Check sheet for the modelled part. Datum: model origin and axes. Units: mm. A direction names the side the tool comes from. Round coordinates to 2 decimals unless told otherwise and drop trailing zeros. Write each loop counter-clockwise with the first axis right and the second up, starting at its lowest first coordinate (ties: lowest second). Pieces come first, ordered by that corner, then holes.
from build123d import *

# Parameters (mm, degrees)
SKETCH_1_R          = 17.4
EXTRUDE_1_DEPTH     = 30
SKETCH_2_R          = 13.5
CUT_EXTRUDE_1_DEPTH = 39.801030914
SKETCH_3_W          = 7.6
SKETCH_3_H          = 1.8
SKETCH_3_W_2        = 1.8
SKETCH_3_H_2        = 7.6
EXTRUDE_2_DEPTH     = 3
SKETCH_4_W          = 20
SKETCH_4_H          = 10
CUT_EXTRUDE_2_DEPTH = 42.164547854
FILLET_1_R          = 5
SKETCH_5_W          = 23.4
SKETCH_5_H          = 23.4
CUT_EXTRUDE_3_DEPTH = 5
FILLET_2_R          = 5


with BuildPart() as part:
    # 草图1 → 凸台-拉伸1 (new body)
    with BuildSketch(Plane(origin=(0, 0, 0), x_dir=(1, 0, 0), z_dir=(0, 1, 0))):
        with Locations(Location((0, 0, 0), (0, 0, 270))):
            Circle(SKETCH_1_R)
    extrude(amount=EXTRUDE_1_DEPTH)

    # 草图2 → 切除-拉伸1 (cut, through all)
    with BuildSketch(Plane(origin=(0, 30, 0), x_dir=(1, 0, 0), z_dir=(0, 1, 0))):
        with Locations(Location((0, 0, 0), (0, 0, 270))):
            Circle(SKETCH_2_R)
    extrude(amount=-CUT_EXTRUDE_1_DEPTH, mode=Mode.SUBTRACT)

    # 草图3 → 凸台-拉伸2 (add)
    with BuildSketch(Plane(origin=(0, 30, 0), x_dir=(1, 0, 0), z_dir=(0, 1, 0))):
        Polygon((13.7, 3.8), (13.7, 0), (13.7, -3.8), (15.5, -3.8), (15.5, 3.8), align=None)
        with Locations((0, -14.6)):
            Rectangle(SKETCH_3_W, SKETCH_3_H)
        with Locations((-14.6, 0)):
            Rectangle(SKETCH_3_W_2, SKETCH_3_H_2)
        with Locations((0, 14.6)):
            Rectangle(SKETCH_3_W, SKETCH_3_H)
    extrude(amount=EXTRUDE_2_DEPTH)

    # 草图4 → 切除-拉伸2 (cut, through all)
    with BuildSketch(Plane(origin=(0, 0, 0), x_dir=(0, 0, -1), z_dir=(1, 0, 0))):
        with Locations((0, 5)):
            Rectangle(SKETCH_4_W, SKETCH_4_H)
    extrude(amount=-CUT_EXTRUDE_2_DEPTH, mode=Mode.SUBTRACT)

    # 圆角1
    fillet_1_edges = [part.edges().sort_by_distance(p)[0] for p in [
        (-11.654280291, 10, -10),
        (-11.654280291, 10, 10),
    ]]
    fillet(fillet_1_edges, radius=FILLET_1_R)

    # 草图5 → 切除-拉伸3 (cut)
    with BuildSketch(Plane(origin=(0, 30, 0), x_dir=(1, 0, 0), z_dir=(0, 1, 0))):
        Rectangle(SKETCH_5_W, SKETCH_5_H)
    extrude(amount=-CUT_EXTRUDE_3_DEPTH, mode=Mode.SUBTRACT)

    # 圆角2
    fillet_2_edges = [part.edges().sort_by_distance(p)[0] for p in [
        (11.7, 27.5, -6.734983296),
        (11.7, 27.5, 6.734983296),
        (6.734983296, 27.5, 11.7),
        (-6.734983296, 27.5, 11.7),
        (-11.7, 27.5, 6.734983296),
        (-11.7, 27.5, -6.734983296),
        (-6.734983296, 27.5, -11.7),
        (6.734983296, 27.5, -11.7),
    ]]
    fillet(fillet_2_edges, radius=FILLET_2_R)


solid = part.part
1. Go/stop test with flat-tipped pins: pin 1 (8 mm diameter, centred on x = 10, y = 3.5, fed in from -Z); pin 2 (10 mm diameter, centred on y = 24, z = 12, fed in from -X); pin 3 (1.4 mm diameter, centred on x = 14.5, y = 32, fed in from +Z); pin 4 (1.9 mm diameter, centred on x = 8, z = 9, fed in from +Y). Record where each tip stops, or that it passes through.
2. Set-up check for faces 1 (the cylindrical face through (-13, 9, 8)), 2 (the flat face through (0, 31, 15.5)), 3 (the flat face through (-15.5, 31, 0)), 4 (the cylindrical face through (-11.827, 27.535, 6.842)): record each of +Z, -Z, +X, -X, +Y, -Y from which the full face is reachable in a straight line by a thin tool's end or side.
3. Sectioned sample at D-D, the plane x = 15. Enter the section's corners in (y, z), plus the area to 3 significant figures.
4. Sectioned sample at C-C, the plane x = 0. Enter the section's corners in (y, z).
5. Scan lines: line 1 along Z through (x, y) = (0, 22.5); line 2 along Z through (x, y) = (12, 18). Record each from-to range of solid material in increasing order.
6. Release check for a two-part mould opening along Z. For faces 5 (the flat face through (0, 31, 13.7)), 6 (the cylindrical face through (17.25, 14.79, -2.27)), 7 (the flat face through (3.8, 31, 15)) record: released by +Z, released by -Z, zero draft, split by the parting line, or undercut.
7. Sectioned sample at B-B, the plane z = 0. Enter the section's corners in (x, y), plus the area to 3 significant figures.
8. Sectioned sample at A-A, the plane y = 26.5. Enter the section's corners in (x, z).
Computed values:
1. pin 1: stops at z = -16.33
1. pin 2: stops at x = -15.93
1. pin 3: stops at z = 3.8
1. pin 4: passes through
2. face 1: -X, -Y
2. face 2: +Z, +X, -X, +Y
2. face 3: +Z, -Z, -X, +Y
2. face 4: +Y
3. outline: (0, -8.82) - (30, -8.82) - (30, -3.8) - (33, -3.8) - (33, 3.8) - (30, 3.8) - (30, 8.82) - (0, 8.82) - close
3. area: 552 mm2
4. outline: (0, -17.4) - (30, -17.4) - (30, -15.5) - (33, -15.5) - (33, -13.7) - (30, -13.7) - (30, -13.5) - (0, -13.5) - close; (0, 13.5) - (30, 13.5) - (30, 13.7) - (33, 13.7) - (33, 15.5) - (30, 15.5) - (30, 17.4) - (0, 17.4) - close
5. line 1: z = -17.4 to -13.5, 13.5 to 17.4
5. line 2: z = -12.6 to -6.18, 6.18 to 12.6
6. face 5: undercut
6. face 6: split by the parting line
6. face 7: zero draft
7. outline: (-17.4, 10) - (-13.5, 10) - (-13.5, 30) - (-13.7, 30) - (-13.7, 33) - (-15.5, 33) - (-15.5, 30) - (-17.4, 30) - close; (13.5, 0) - (17.4, 0) - (17.4, 30) - (15.5, 30) - (15.5, 33) - (13.7, 33) - (13.7, 30) - (13.5, 30) - close
7. area: 206 mm2
8. outline: circle Ø34.8 at (0, 0); hole (-12.19, -5.81) arc R5 cw to (-11.7, -7.96) - (-11.7, -11.7) - (-7.96, -11.7) arc R5 cw to (-5.81, -12.19) arc R13.5 ccw to (5.81, -12.19) arc R5 cw to (7.96, -11.7) - (11.7, -11.7) - (11.7, -7.96) arc R5 cw to (12.19, -5.81) arc R13.5 ccw to (12.19, 5.81) arc R5 cw to (11.7, 7.96) - (11.7, 11.7) - (7.96, 11.7) arc R5 cw to (5.81, 12.19) arc R13.5 ccw to (-5.81, 12.19) arc R5 cw to (-7.96, 11.7) - (-11.7, 11.7) - (-11.7, 7.96) arc R5 cw to (-12.19, 5.81) arc R13.5 ccw to start
